```python
from build123d import *

# Parameters (mm, degrees)
F1_DEPTH     = 1.55
F3_DEPTH     = 0.35
F4_W         = 8.65
F4_H         = 1
F5_DEPTH     = 1.3
F7_W         = 4.25
F7_H         = 4
F8_DEPTH     = 2.55
F10_DEPTH    = 39.5010001
F11_W        = 4
F11_H        = 1.275
F12_DEPTH    = 1.1
F13_W        = 8.65
F13_H        = 1
F14_DEPTH    = 1.4
F15_DEPTH    = 38.0010001
F17_DEPTH    = 1.4
F18_T4_DEPTH = 11.4290603676
F19_T4_DEPTH = 10.6517870966
F20_W        = 1.4
F20_H        = 3.8
F21_DEPTH    = 2.2
F22_W        = 3.8
F22_H        = 1.1
F23_DEPTH    = 0.5
F24_R        = 0.5


# Not quite as in the source:
# - a fillet or chamfer that OpenCascade refuses, or shapes differently, is made with other operations: its cross-section is extruded or revolved along the edge and cut away or added


with BuildPart() as f1:
    # F0 (on Top) → F1 (new body)
    with BuildSketch(Plane.XY):
        with BuildLine():
            Line((-12.4797472133, -24.9172599055), (1.8202527867, -24.9172599055))
            ThreePointArc((1.8202527867, -24.9172599055), (3.9415731303, -24.038580249), (4.8202527867, -21.9172599055))
            Line((4.8202527867, -21.9172599055), (4.8202527867, 20.0827400945))
            ThreePointArc((4.8202527867, 20.0827400945), (3.9415731303, 22.2040604381), (1.8202527867, 23.0827400945))
            Line((1.8202527867, 23.0827400945), (-5.1797472133, 23.0827400945))
            ThreePointArc((-5.1797472133, 23.0827400945), (-7.3010675568, 22.2040604381), (-8.1797472133, 20.0827400945))
            Line((-8.1797472133, 20.0827400945), (-8.1797472133, 10.0827400945))
            add(Edge.make_bspline(
                [(-8.1797472133, 10.0827400945), (-8.4297074571, 7.300546721), (-9.1785947804, 5.6351239407), (-11.0454632546, 3.7753203501), (-12.7602456599, 2.4755173938), (-13.6481305175, 1.4367913649), (-14.42578763, 0.9165801451)],
                knots=[0, 0, 0, 0, 0.3064186573, 0.5153311453, 0.7233584291, 0.9057268673, 0.9057268673, 0.9057268673, 0.9057268673], degree=3))
            ThreePointArc((-14.42578763, 0.9165801451), (-15.5669094587, -0.3434616219), (-15.9797472133, -1.9925308353))
            Line((-15.9797472133, -1.9925308353), (-15.9797472133, -21.4172599055))
            ThreePointArc((-15.9797472133, -21.4172599055), (-14.9546209474, -23.8921336396), (-12.4797472133, -24.9172599055))
        make_face()
        with BuildLine():
            Line((-14.5797472133, -21.3672599055), (-14.5797472133, -3.1172599055))
            ThreePointArc((-14.5797472133, -3.1172599055), (-14.3747219601, -2.6222851587), (-13.8797472133, -2.4172599055))
            ThreePointArc((-13.8797472133, -2.4172599055), (-13.3847724664, -2.6222851587), (-13.1797472133, -3.1172599055))
            Line((-13.1797472133, -3.1172599055), (-13.1797472133, -21.3672599055))
            ThreePointArc((-13.1797472133, -21.3672599055), (-13.3847724664, -21.8622346523), (-13.8797472133, -22.0672599055))
            ThreePointArc((-13.8797472133, -22.0672599055), (-14.3747219601, -21.8622346523), (-14.5797472133, -21.3672599055))
        make_face(mode=Mode.SUBTRACT)
    extrude(amount=F1_DEPTH)

    # F2 (on face) → F3 (join)
    with BuildSketch(Plane.XY.offset(1.55)):
        with BuildLine():
            Line((1.5702527867, 21.0827400945), (-4.6797472133, 21.0827400945))
            ThreePointArc((-4.6797472133, 21.0827400945), (-6.0939607756, 20.4969536569), (-6.6797472133, 19.0827400945))
            Line((-6.6797472133, 19.0827400945), (-6.6797472133, -22.9172599055))
            Line((-6.6797472133, -22.9172599055), (1.5702527867, -22.9172599055))
            ThreePointArc((1.5702527867, -22.9172599055), (2.9844663491, -22.3314734679), (3.5702527867, -20.9172599055))
            Line((3.5702527867, -20.9172599055), (3.5702527867, 19.0827400945))
            ThreePointArc((3.5702527867, 19.0827400945), (2.9844663491, 20.4969536569), (1.5702527867, 21.0827400945))
        make_face()
    extrude(amount=F3_DEPTH)

    # F4 (on face) → F5 (join)
    with BuildSketch(Plane.XY.offset(1.9)):
        with Locations((-1.7547472133, 13.5827400945)):
            Rectangle(F4_W, F4_H)
        with Locations((-1.7547472133, -14.4172599055)):
            Rectangle(F4_W, F4_H)
    extrude(amount=F5_DEPTH)

    # F7 (on face) → F8 (join)
    with BuildSketch(Plane.XY.offset(1.55)):
        with Locations((2.6952527867, -14.4172599055)):
            Rectangle(F7_W, F7_H)
        with Locations((2.6952527867, 13.5827400945)):
            Rectangle(F7_W, F7_H)
    extrude(amount=F8_DEPTH)

    # F9 (on face) → F10 (cut, through all)
    with BuildSketch(Plane.XZ.offset(16.4172599055)):
        with BuildLine():
            Line((0.5702527867, 4.1), (0.5702527867, 1.9))
            ThreePointArc((0.5702527867, 1.9), (1.620780987, 2.8944421952), (2.4202527867, 4.1))
            Line((2.4202527867, 4.1), (0.5702527867, 4.1))
        make_face()
    extrude(amount=-F10_DEPTH, mode=Mode.SUBTRACT)

    # F11 (on face) → F12 (join)
    with BuildSketch(Plane.YZ.offset(4.8202527867)):
        with Locations((-14.4172599055, 3.4625)):
            Rectangle(F11_W, F11_H)
        with Locations((13.5827400945, 3.4625)):
            Rectangle(F11_W, F11_H)
    extrude(amount=F12_DEPTH)

    # F13 (on face) → F14 (join)
    with BuildSketch(Plane.XY.offset(1.9)):
        with Locations((-1.7547472133, -14.4172599055)):
            Rectangle(F13_W, F13_H)
        with Locations((-1.7547472133, 13.5827400945)):
            Rectangle(F13_W, F13_H)
    extrude(amount=F14_DEPTH)

    # F6 (on face) → F15 (cut, through all)
    with BuildSketch(Plane.XZ.offset(14.9172599055)):
        with BuildLine():
            Line((1.6002527867, 3.2), (-5.1997472133, 3.2))
            ThreePointArc((-5.1997472133, 3.2), (-1.7997472133, 2), (1.6002527867, 3.2))
        make_face()
        with BuildLine():
            ThreePointArc((3.6169194534, 7.4166666667), (-4.1367978237, 12.3032270339), (-5.1997472133, 3.2))
            Line((-5.1997472133, 3.2), (1.6002527867, 3.2))
            ThreePointArc((1.6002527867, 3.2), (3.0868131539, 5.0796160563), (3.6169194534, 7.4166666667))
        make_face()
    extrude(amount=-F15_DEPTH, mode=Mode.SUBTRACT)

    # F16 (on face) → F17 (cut)
    with BuildSketch(Plane.XY.offset(1.9)):
        Polygon((-6.6797472133, -22.9172599055), (-6.6797472133, -5.2834198549), (-13.1797472133, -5.2834198549), (-13.7797472133, -5.2834198549), (-13.7797472133, -23.7172599055), (-6.2646348961, -23.7172599055), (-6.2646348961, -22.9172599055), align=None)
    extrude(amount=-F17_DEPTH, mode=Mode.SUBTRACT)

    # F18: chamfer of 1.1 x 1.9052558883 on 1 edges, made by hand


with BuildPart() as f18_tool2:
    # F18_s3 → F18_t4 (new body)
    with BuildSketch(Plane.YZ.offset(-1.7506868456)):
        Polygon((-7.1886757432, 0.5), (-5.2834198549, 1.6), (-5.2834198549, 0.5), align=None)
    extrude(amount=-F18_T4_DEPTH)

    split(bisect_by=Plane.XY.offset(1.55), keep=Keep.BOTTOM)


with BuildPart() as f1_1:
    add(f1.part)

    # F18_t1: union F18_tool2
    add(f18_tool2.part)

    # F19: chamfer of 0.7 x 1.2124355653 on 1 edges, made by hand


with BuildPart() as f19_tool2:
    # F19_s3 → F19_t4 (new body)
    with BuildSketch(Plane.YZ.offset(-13.7797472133)):
        Polygon((-23.0172599055, 0.5), (-23.7172599055, 1.7124355653), (-23.7172599055, 0.5), align=None)
    extrude(amount=F19_T4_DEPTH)

    split(bisect_by=Plane.XY.offset(1.55), keep=Keep.BOTTOM)


with BuildPart() as f1_2:
    add(f1_1.part)

    # F19_t1: union F19_tool2
    add(f19_tool2.part)

    # F20 (on face) → F21 (join)
    with BuildSketch(Plane.XY.offset(1.55)):
        with Locations((-15.2797472133, -11.4172599055)):
            Rectangle(F20_W, F20_H)
    extrude(amount=F21_DEPTH)

    # F22 (on face) → F23 (join)
    with BuildSketch(Plane(origin=(-15.9797472133, 0, 0), x_dir=(0, -1, 0), z_dir=(-1, 0, 0))):
        with Locations((11.4172599055, 3.2)):
            Rectangle(F22_W, F22_H)
    extrude(amount=F23_DEPTH)

    # F24
    f24_edges = [f1_2.edges().sort_by_distance(p)[0] for p in [
        (-15.279747, -13.31726, 1.55),
        (-15.279747, -9.51726, 1.55),
        (-16.479747, -11.41726, 3.75),
    ]]
    fillet(f24_edges, radius=F24_R)


solid = f1_2.part
```
Design review of the part built by this model. Coordinates are the model's own, in mm. A direction names the side the tool comes from. Give positions to 0.01 mm unless a question says otherwise; leave off trailing zeros. Write each loop counter-clockwise with the first axis right and the second up, starting at its lowest first coordinate (ties: lowest second). Pieces come first, ordered by that corner, then holes.
(1) Tool access review of faces 1 (the face through (-9.88, -6.29, 1.02)), 2 (the face through (5, -14, 2.825)), 3 (the face through (-14.58, -12, 1)), 4 (the face through (4, 0, 1.55)), 5 (the face through (2.969, -22.347, 1.723)): name each direction out of +Z, -Z, +X, -X, +Y, -Y from which nothing blocks a thin tool from reaching the whole face with its end or side.
Checked values:
face 1: +Z
face 2: -Z, +X, +Y, -Y
face 3: +Z, -Z
face 4: +Z, +X
face 5: +Z, +X, -Y
(2) Wall thickness on line 1 along X through (y, z) = (-12.5, 1.35); line 2 along Y through (x, z) = (3.5, 3.5); line 3 along Z through (x, y) = (4.5, 21): over which ranges is each line inside the solid? List them lowest first.
Checked values:
line 1: x = -15.98 to -14.58, -6.68 to 4.82
line 2: y = -16.42 to -12.42, 11.58 to 15.58
line 3: z = 0 to 1.55
(3) Add section A-A (y = -15.5). Give the boundary of the cut face in (x, z) (3 decimals), and give its area (3 significant figures).
Checked values:
outline: (-15.98, 0) - (-14.58, 0) - (-14.58, 1.55) - (-15.98, 1.55) - close; (-13.18, 0) - (4.82, 0) - (4.82, 2.825) - (5.92, 2.825) - (5.92, 4.1) - (2.42, 4.1) arc R6.379 cw to (0.57, 1.9) - (-6.68, 1.9) - (-6.68, 0.5) - (-13.18, 0.5) - close
area: 35.7 mm2
(4) Clearance check with flat-ended pins moving along their axes: pin 1 Ø1 at (x, y) = (-9, 17.5) entering from +Z; pin 2 Ø0.8 at (x, z) = (3.5, 2.5) entering from +Y; pin 3 Ø1.1 at (x, z) = (-4, 2.5) entering from +Y; pin 4 Ø8 at (x, y) = (-3, -2.5) entering from +Z. State where each tip first meets the part, or that it passes through.
Checked values:
pin 1: passes through
pin 2: stops at y = 15.58
pin 3: stops at y = 14.08
pin 4: stops at z = 1.9
(5) Add section B-B (y = 16.5). Give the boundary of the cut face in (x, z), and give its area (3 significant figures).
Checked values:
outline: (-8.18, 0) - (4.82, 0) - (4.82, 1.55) - (3.57, 1.55) - (3.57, 1.9) - (-6.68, 1.9) - (-6.68, 1.55) - (-8.18, 1.55) - close
area: 23.7 mm2
(6) Mouldability with a two-part tool opening along Y and no side actions: class faces 6 (the face through (-3.9, -13.917, 2.1)), 7 (the face through (-4.9, -23.5, 1.55)), 8 (the face through (-14.982, -23.865, 0.764)) as +Y half, -Y half, draft (parallel to the pull), parting line (faces both ways), or undercut.
Checked values:
face 6: undercut
face 7: draft
face 8: -Y half
(7) Add section C-C (x = -3.5). Give the boundary of the cut face in (y, z).
Checked values:
outline: (-24.92, 0) - (23.08, 0) - (23.08, 1.55) - (21.08, 1.55) - (21.08, 1.9) - (14.08, 1.9) - (14.08, 2.27) - (13.08, 2.27) - (13.08, 1.9) - (-13.92, 1.9) - (-13.92, 2.27) - (-14.92, 2.27) - (-14.92, 1.9) - (-22.92, 1.9) - (-22.92, 1.55) - (-24.92, 1.55) - close
